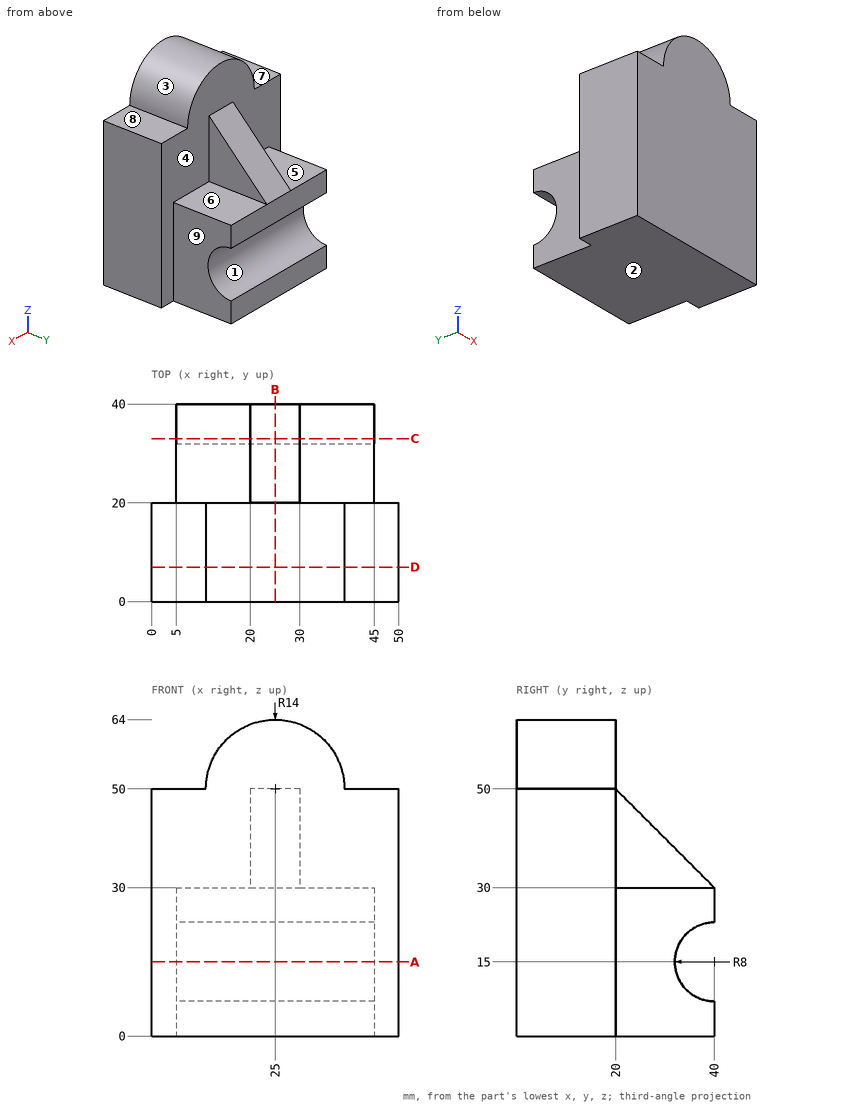
Drawing for the job (mm, zero at the part's lowest x, y, z). A direction names the side the tool comes from. Round coordinates to 2 decimals unless told otherwise and drop trailing zeros. Write each loop counter-clockwise with the first axis right and the second up, starting at its lowest first coordinate (ties: lowest second). Pieces come first, ordered by that corner, then holes. Notation, with made-up numbers: M -33.5,31.25 L 20.5,31.25 A27 cw 20.5,52.25 Z; hole C 29.5,-35 d6. An arc over 180 degrees is marked long. One line per question, with ' | ' between items.
1. Pin check, flat tips, straight feed: pin 1 Ø1.5 at (y, z) = (34, 30) entering from -X; pin 2 Ø7.5 at (x, y) = (38, 25.5) entering from +Z; pin 3 Ø9 at (x, y) = (6, 7) entering from +Z. Stop position of each tip, or through.
Working result:
pin 1: x = 5 | pin 2: z = 30 | pin 3: z = 50
2. Cut at A-A on z = 15. Write the cut outline in (x, y).
Working result:
outline: M 0,0 L 50,0 L 50,20 L 45,20 L 45,32 L 5,32 L 5,20 L 0,20 Z
3. Cut at B-B on x = 25. Write the cut outline in (y, z).
Working result:
outline: M 0,0 L 40,0 L 40,7 A8 cw 40,23 L 40,30 L 20,50 L 20,64 L 0,64 Z
4. Probe L1, parallel to Y at x = 35, z = 31; L2, parallel to X at y = 26.5, z = 24.5; L3, parallel to Z at x = 7, y = 11. List the from-to ranges inside material, lowest first. Write a range as from..to.
Working result:
L1: 0..20 | L2: 5..45 | L3: 0..50
5. Mould opens along Z. For the marked faces 1, 2, 3 and 4 say: pulls with the +Z half, pulls with the -Z half, needs draft (parallel to the pull), parting line crosses it, or undercut.
Working result:
face 1: undercut | face 2: pulls with the -Z half | face 3: pulls with the +Z half | face 4: needs draft
6. Cut at D-D on y = 7. Write the cut outline in (x, z).
Working result:
outline: M 0,0 L 50,0 L 50,50 L 39,50 A14 ccw 11,50 L 0,50 Z
7. Which spindle directions (+Z, -Z, +X, -X, +Y, -Y) get a long thin tool onto all of the face, cutting with end or side? Do the marked faces 5, 6, 7, 8 and 9. Say none if no direction does.
Working result:
face 5: +Z, -X, +Y | face 6: +Z, +X, +Y | face 7: +Z, -X, +Y, -Y | face 8: +Z, +X, +Y, -Y | face 9: +Z, -Z, +X, +Y
8. Cut at C-C on y = 33. Write the cut outline in (x, z).
Working result:
outline: M 5,0 L 45,0 L 45,11.13 L 5,11.13 Z; M 5,18.87 L 45,18.87 L 45,30 L 30,30 L 30,37 L 20,37 L 20,30 L 5,30 Z
